```python
from build123d import *

# Parameters (mm, degrees)
F0_R      = 36.0888023615
F0_R_2    = 29.21
F1_DEPTH  = 50.8
F2_R      = 36.0888023615
F3_DEPTH  = 6.35
F6_R      = 22.8868793225
F6_R_2    = 18.2059808832
F7_DEPTH  = 96.52
F8_DEPTH  = 76.2
F10_D     = 58.42
F10_DEPTH = 101.6
F10_TIP   = 17.5511386818
F11_R     = 32.1245501008
F11_R_2   = 22.8868793225
F11_R_3   = 18.2059808832
F12_DEPTH = 6.35
F14_D     = 10.16
F15_R     = 12.7


with BuildPart() as f1:
    # F0 (on Top) → F1 (new body)
    with BuildSketch(Plane.XY):
        Circle(F0_R)
        Circle(F0_R_2, mode=Mode.SUBTRACT)
    extrude(amount=F1_DEPTH)


with BuildPart() as f3:
    # F2 (on face) → F3 (new body)
    with BuildSketch(Plane.XY.offset(50.8)):
        Polygon((63.5, 63.5), (0, 63.5), (-63.5, 63.5), (-63.5, 0), (-63.5, -63.5), (0, -63.5), (63.5, -63.5), (63.5, 0), align=None)
        Circle(F2_R, mode=Mode.SUBTRACT)
    extrude(amount=-F3_DEPTH)

    # F4: union F1
    add(f1.part)

    # F5: F3 across plane


with BuildPart() as f3_1:
    add(f3.part)
    add(f3.part.mirror(Plane.XY))

    # F6 (on Front) → F7 (join)
    with BuildSketch(Plane.XZ):
        Circle(F6_R)
        Circle(F6_R_2, mode=Mode.SUBTRACT)
    extrude(amount=F7_DEPTH)

    # F6 (on Front) → F8 (cut)
    with BuildSketch(Plane.XZ):
        Circle(F6_R_2)
    extrude(amount=F8_DEPTH, mode=Mode.SUBTRACT)

    # F10
    with Locations(Plane.XY.offset(50.8)):
        with Locations((0, 0)):
            Hole(F10_D / 2, depth=F10_DEPTH)
            with Locations((0, 0, -(F10_DEPTH + F10_TIP / 2))):  # 118° drill point
                Cone(0, F10_D / 2, F10_TIP, mode=Mode.SUBTRACT)

    # F11 (on face) → F12 (join)
    with BuildSketch(Plane.XZ.offset(96.52)):
        Circle(F11_R)
        Circle(F11_R_2, mode=Mode.SUBTRACT)
        Circle(F11_R_2)
        Circle(F11_R_3, mode=Mode.SUBTRACT)
    extrude(amount=-F12_DEPTH)

    # F14 (through all)
    with Locations(Plane.XY.offset(50.8)):
        with Locations((53.34, 53.34), (53.34, -53.34), (-53.34, -53.34), (-53.34, 53.34)):
            Hole(F14_D / 2)

    # F15
    f15_edges = [f3_1.edges().sort_by_distance(p)[0] for p in [
        (-63.5, 63.5, -47.625),
        (-63.5, 63.5, 47.625),
        (-63.5, -63.5, -47.625),
        (-63.5, -63.5, 47.625),
        (63.5, -63.5, 47.625),
        (63.5, -63.5, -47.625),
        (63.5, 63.5, 47.625),
        (63.5, 63.5, -47.625),
    ]]
    fillet(f15_edges, radius=F15_R)


solid = f3_1.part
```
Read the model definition and answer for the solid it produces. Units are mm, in the model's axes. A direction names the side the tool comes from. Give positions to 0.01 mm unless a question says otherwise; leave off trailing zeros. Loops run counter-clockwise (first coordinate to the right, second up) from the corner with the lowest first, then second, coordinate; pieces in that order, holes last.
Item 1: Each of these flat-tipped pins is pushed along its axis until it touches: pin 1 Ø6 at (x, y) = (53.34, -53.34) entering from -Z; pin 2 Ø6 at (y, z) = (-19.5, 13) entering from +X; pin 3 Ø8 at (x, z) = (36.5, -21.5) entering from +Y; pin 4 Ø7 at (x, z) = (-8, 49) entering from -Y. Where does it stop, or does it pass through?
Item 2: The part is cut by section B-B (y = 0). Write down the section's boundary in (x, z).
Item 3: The mould has two halves that part along Y. Classify faces 1 (the cylindrical face through (59.88, -59.68, -47.58)), 2 (the flat face through (1, 63.5, -48)), 3 (the flat face through (-8, -90.17, 22)): released by +Y, released by -Y, zero draft, split by the parting line, or undercut.
Item 4: The part is cut by section D-D (z = 25). Write down the section's boundary in (x, y), and give its area (3 significant figures).
Item 5: For faces 4 (the cylindrical face through (-18.19, -59.16, 0.8)), 5 (the cylindrical face through (-4.7, 35.78, -0.62)), 6 (the flat face through (-1, -63.5, -48)), determine the directions among +Z, -Z, +X, -X, +Y, -Y from which every point of the face is accessible in a straight line to the end or side of a thin tool.
Item 6: The part is cut by section C-C (x = 0). Write down the section's boundary in (y, z).
Item 7: The part is cut by section A-A (y = -45.5). Write down the section's boundary in (x, z), and give its area (3 significant figures).
Item 8: Find the intervals of material crossed by line 1 along Z through (x, y) = (39, -25); line 2 along Y through (x, z) = (53, -48); line 3 along Z through (x, y) = (5, -53), in increasing order.
Taken from the geometry:
1. pin 1: passes through
1. pin 2: stops at x = 32.1
1. pin 3: stops at y = 15.69
1. pin 4: stops at y = -63.5
2. outline: (-63.5, -50.8) - (-29.21, -50.8) - (-29.21, 50.8) - (-63.5, 50.8) - (-63.5, 44.45) - (-36.09, 44.45) - (-36.09, -44.45) - (-63.5, -44.45) - close; (29.21, -50.8) - (63.5, -50.8) - (63.5, -44.45) - (36.09, -44.45) - (36.09, 44.45) - (63.5, 44.45) - (63.5, 50.8) - (29.21, 50.8) - close
3. face 1: released by -Y
3. face 2: released by +Y
3. face 3: undercut
4. outline: circle Ø72.18 at (0, 0); (-20.17, -96.52) - (20.17, -96.52) - (20.17, -90.17) - (-20.17, -90.17) - close; hole circle Ø58.42 at (0, 0)
4. area: 1,670 mm2
5. face 4: -Y
5. face 5: none
5. face 6: -Z, +X, -X, -Y
6. outline: (-96.52, -32.12) - (-90.17, -32.12) - (-90.17, -22.89) - (-36.09, -22.89) - (-36.09, -44.45) - (-63.5, -44.45) - (-63.5, -50.8) - (-29.21, -50.8) - (-29.21, -18.21) - (-96.52, -18.21) - close; (-96.52, 18.21) - (-29.21, 18.21) - (-29.21, 50.8) - (-63.5, 50.8) - (-63.5, 44.45) - (-36.09, 44.45) - (-36.09, 22.89) - (-90.17, 22.89) - (-90.17, 32.12) - (-96.52, 32.12) - close; (29.21, -50.8) - (63.5, -50.8) - (63.5, -44.45) - (36.09, -44.45) - (36.09, 44.45) - (63.5, 44.45) - (63.5, 50.8) - (29.21, 50.8) - close
7. outline: (-63.5, -50.8) - (63.5, -50.8) - (63.5, -44.45) - (-63.5, -44.45) - close; (-63.5, 44.45) - (63.5, 44.45) - (63.5, 50.8) - (-63.5, 50.8) - close; circle Ø45.77 at (0, 0); hole circle Ø36.41 at (0, 0)
7. area: 2,220 mm2
8. line 1: z = -50.8 to -44.45, 44.45 to 50.8
8. line 2: y = -63.31 to -58.41, -48.27 to 48.27, 58.41 to 63.31
8. line 3: z = -50.8 to -44.45, -22.33 to -17.51, 17.51 to 22.33, 44.45 to 50.8
